from build123d import *

# Parameters (mm, degrees)
ESBO_O2_R             = 3
CORTE_EXTRUS_O1_DEPTH = 7


with BuildPart() as part:
    # Esboço1 → Revolução1 (revolve)
    with BuildSketch(Plane.XY):
        Polygon((0, 23), (0, 42.5), (6, 42.5), (6, 30), (20, 30), (20, 20), (15, 20), (15, 22), (3, 22), (3, 24.5), (1.5, 24.5), (1.5, 23), align=None)
    revolve(axis=Axis((0, 0, 0), (1, 0, 0)))

    # Esboço2 → Corte-extrusão1 (cut, through all)
    with BuildSketch(Plane(origin=(6, 0, 0), x_dir=(0, 0, -1), z_dir=(1, 0, 0))):
        with Locations((0, 36.25)):
            Circle(ESBO_O2_R)
        with Locations((36.25, 0)):
            Circle(ESBO_O2_R)
        with Locations((0, -36.25)):
            Circle(ESBO_O2_R)
        with Locations((-36.25, 0)):
            Circle(ESBO_O2_R)
    extrude(amount=-CORTE_EXTRUS_O1_DEPTH, mode=Mode.SUBTRACT)


solid = part.part
Can you work these out from the model? Positions are in its coordinate system, mm. A direction names the side the tool comes from. Round coordinates to 2 decimals unless told otherwise and drop trailing zeros. Write each loop counter-clockwise with the first axis right and the second up, starting at its lowest first coordinate (ties: lowest second). Pieces come first, ordered by that corner, then holes. Notation, with made-up numbers: (-27, 69) - (-4, 69) arc R6 cw to (-4, 78) - close; hole circle Ø9 at (77.5, 37.5). An arc over 180 degrees is marked (long way). Write each question's results on one line, items separated by ' | '. Start each with the question number.
1) We'd pull the mould along Y, two halves only. Please class faces 1 (the flat face through (15, -10, -18)), 2 (the cylindrical face through (13.1, -29.97, 1.32)), 3 (the flat face through (20, 6, -20)): released by +Y, released by -Y, zero draft, split by the parting line, or undercut.
2) Suppose I cut it at C-C (x = 5). List the corners of the cut face in (y, z) for me, and give its area (3 significant figures).
3) Suppose I cut it at A-A (y = 0). Give the number of separate pieces and of enclosed holes in the cut face, and give its area (4 significant figures).
4) For pin 1 Ø1.5 at (x, y) = (12, -25.5) entering from +Z; pin 2 Ø12 at (x, y) = (8, -1.5) entering from -Z; pin 3 Ø2 at (x, z) = (11, 19) entering from -Y, each with a flat end and sliding along its axis, tell me the tip position at first contact or that it passes through.
5) Suppose I cut it at D-D (z = 36.25). List the corners of the cut face in (x, y) for me.
6) Please list where these lines run through material, in increasing order: line 1 (Z direction, x = 17.6, y = 0); line 2 (Z direction, x = 12.5, y = 0); line 3 (Y direction, x = 3.25, z = 2).
7) Which directions (+Z, -Z, +X, -X, +Y, -Y) give clear straight access to the entire face, cutting with the end or side of a thin tool? Please do faces 4 (the flat face through (6, -10, 29)), 5 (the cylindrical face through (8.916, -4.769, -21.477)), 6 (the flat face through (3, 18, 13)).
Here are the results:
1) face 1: undercut | face 2: split by the parting line | face 3: zero draft
2) outline: circle Ø85 at (0, 0); hole circle Ø6 at (-36.25, 0); hole circle Ø44 at (0, 0); hole circle Ø6 at (0, -36.25); hole circle Ø6 at (0, 36.25); hole circle Ø6 at (36.25, 0) | area: 4,040 mm2
3) separate pieces: 4 | enclosed holes: 0 | area: 407.5 mm2
4) pin 1: stops at z = 16.95 | pin 2: stops at z = -42.5 | pin 3: stops at y = -24
5) outline: (0, -22.19) - (6, -22.19) - (6, -3) - (0, -3) - close; (0, 3) - (6, 3) - (6, 22.19) - (0, 22.19) - close
6) line 1: z = -30 to -20, 20 to 30 | line 2: z = -30 to -22, 22 to 30 | line 3: y = -42.45 to -38.49, -34.01 to -21.91, 21.91 to 34.01, 38.49 to 42.45
7) face 4: +X | face 5: -X | face 6: none
